CAD build for the part. Positions are in the model's coordinates, mm. Face numbers are marked on the shaded views. A direction names the side the tool comes from. Coordinates: 2 decimals unless noted, no trailing zeros. Loops run counter-clockwise (first coordinate to the right, second up) from the corner with the lowest first, then second, coordinate; pieces in that order, holes last. Notation, with made-up numbers: (-7.75, 6.5) -> (44.25, 6.5) arc R16 cw to (44.25, 31.5) -> close; hole circle Ø10 at (13, 14.5). An arc over 180 degrees is marked (long way). Write each question's results on one line, items separated by ' | '.
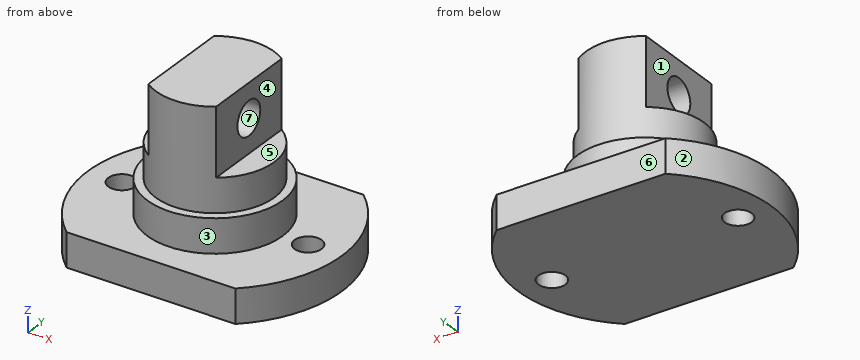
from build123d import *

# Parameters (mm, degrees)
F1_DEPTH  = 10
F2_R      = 4
F3_DEPTH  = 10
F4_R      = 20
F5_DEPTH  = 10
F6_R      = 17.5
F7_DEPTH  = 30
F9_DEPTH  = 20
F10_R     = 5
F11_DEPTH = 20


with BuildPart() as f1:
    # F0 (on Top) → F1 (new body)
    with BuildSketch(Plane.XY):
        with BuildLine():
            Line((24.944939, 28), (-24.944939, 28))
            ThreePointArc((-24.944939, 28), (-37.5, 0), (-24.944939, -28))
            Line((-24.944939, -28), (24.944939, -28))
            ThreePointArc((24.944939, -28), (37.5, 0), (24.944939, 28))
        make_face()
    extrude(amount=F1_DEPTH)

    # F2 (on face) → F3 (cut, through all)
    with BuildSketch(Plane.XY.offset(10)):
        with Locations((-27.5, 0)):
            Circle(F2_R)
        with Locations((27.5, 0)):
            Circle(F2_R)
    extrude(amount=-F3_DEPTH, mode=Mode.SUBTRACT)

    # F4 (on face) → F5 (join)
    with BuildSketch(Plane.XY.offset(10)):
        Circle(F4_R)
    extrude(amount=F5_DEPTH)

    # F6 (on face) → F7 (join)
    with BuildSketch(Plane.XY.offset(20)):
        Circle(F6_R)
    extrude(amount=F7_DEPTH)

    # F8 (on face) → F9 (cut)
    with BuildSketch(Plane.XY.offset(50)):
        with BuildLine():
            Line((-10, -14.361407), (-10, 14.361407))
            ThreePointArc((-10, 14.361407), (-17.5, 0), (-10, -14.361407))
        make_face()
        with BuildLine():
            ThreePointArc((17.5, 0), (15.512092, 8.100926), (10, 14.361407))
            Line((10, 14.361407), (10, -14.361407))
            ThreePointArc((10, -14.361407), (15.512092, -8.100926), (17.5, 0))
        make_face()
    extrude(amount=-F9_DEPTH, mode=Mode.SUBTRACT)

    # F10 (on face) → F11 (cut, through all)
    with BuildSketch(Plane.YZ.offset(10)):
        with Locations((0, 40)):
            Circle(F10_R)
    extrude(amount=-F11_DEPTH, mode=Mode.SUBTRACT)


solid = f1.part
1) Slice it at B-B (x = 0). Write the cut outline in (y, z), then the cut area to 3 significant figures.
Outcome:
outline: (-28, 0) -> (28, 0) -> (28, 10) -> (20, 10) -> (20, 20) -> (17.5, 20) -> (17.5, 50) -> (-17.5, 50) -> (-17.5, 20) -> (-20, 20) -> (-20, 10) -> (-28, 10) -> close; hole circle Ø10 at (0, 40) | area: 1,930 mm^2
2) Drill centre lines: L1, parallel to Z at x = -2.25, y = 0; L2, parallel to Z at x = 13, y = -16; L3, parallel to X at y = -13, z = 46. Where is each one in solid material? Low to high. Write a range as from..to.
Outcome:
L1: z = 0..35, 45..50 | L2: z = 0..10 | L3: x = -10..10
3) Pin check, flat tips, straight feed: pin 1 (6 mm diameter, centred on x = -1, z = 35, fed in from +Y); pin 2 (3 mm diameter, centred on x = 7, z = 43, fed in from +Y); pin 3 (3 mm diameter, centred on x = -16, y = -2, fed in from +Z). Stop position of each tip, or through.
Outcome:
pin 1: stops at y = 17.5 | pin 2: stops at y = 16.61 | pin 3: stops at z = 30
4) Slice it at C-C (y = 0). Write the cut outline in (x, z).
Outcome:
outline: (-37.5, 0) -> (-31.5, 0) -> (-31.5, 10) -> (-37.5, 10) -> close; (-23.5, 0) -> (23.5, 0) -> (23.5, 10) -> (20, 10) -> (20, 20) -> (17.5, 20) -> (17.5, 30) -> (10, 30) -> (10, 35) -> (-10, 35) -> (-10, 30) -> (-17.5, 30) -> (-17.5, 20) -> (-20, 20) -> (-20, 10) -> (-23.5, 10) -> close; (-10, 45) -> (10, 45) -> (10, 50) -> (-10, 50) -> close; (31.5, 0) -> (37.5, 0) -> (37.5, 10) -> (31.5, 10) -> close
5) Which spindle directions (+Z, -Z, +X, -X, +Y, -Y) get a long thin tool onto all of the face, cutting with end or side? Do the marked faces 1, 2, 3 and 4. Say none if no direction does.
Outcome:
face 1: +Z, -X, +Y, -Y | face 2: +Z, -Z, -X | face 3: +Z | face 4: +Z, +X, +Y, -Y
6) Slice it at D-D (z = 3.5). Write the cut outline in (x, y), then the cut area to 3 significant figures.
Outcome:
outline: (-24.94, -28) -> (24.94, -28) arc R37.5 ccw to (24.94, 28) -> (-24.94, 28) arc R37.5 ccw to start; hole circle Ø8 at (-27.5, 0); hole circle Ø8 at (27.5, 0) | area: 3,670 mm^2
7) Two-plate mould, pull along Z, no slides. Class the marked faces 5, 6 and 7: pulls with the +Z half, pulls with the -Z half, needs draft (parallel to the pull), parting line crosses it, or undercut.
Outcome:
face 5: pulls with the +Z half | face 6: needs draft | face 7: undercut
8) Slice it at A-A (z = 40). Write the cut outline in (x, y).
Outcome:
outline: (-10, -14.36) arc R17.5 ccw to (10, -14.36) -> (10, -5) -> (-10, -5) -> close; (-10, 5) -> (10, 5) -> (10, 14.36) arc R17.5 ccw to (-10, 14.36) -> close
